Part model, mm, in its own coordinate system. Face numbers are marked on the shaded views. A direction names the side the tool comes from. Give positions to 0.01 mm unless a question says otherwise; leave off trailing zeros. Order: outer loops, then holes, each group sorted by start corner. A loop starts at its lowest first (then second) coordinate and runs counter-clockwise, first axis right, second up. Notation, with made-up numbers: M 67,25 L 104,25 A23 ccw 104,46 Z; hole C 82.5,57.5 d11. An arc over 180 degrees is marked long. Return JSON: item names as keys, results as strings.
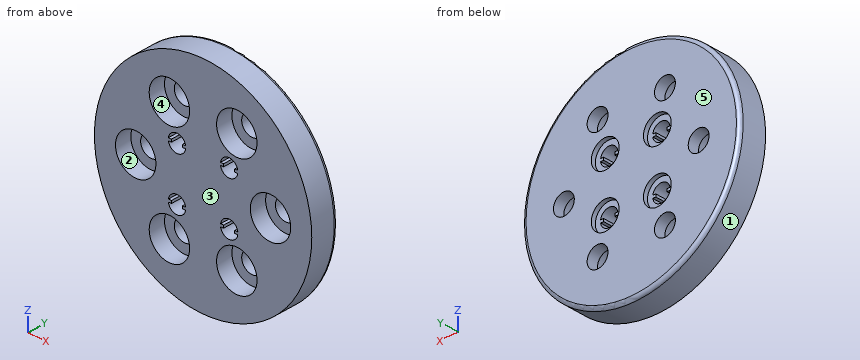
from build123d import *

# Parameters (mm, degrees)
SKETCH1_R           = 25
BOSS_EXTRUDE1_DEPTH = 6.35
SKETCH3_R           = 2.4
CUT_EXTRUDE3_DEPTH  = 7.35
SKETCH4_R           = 4.65
CUT_EXTRUDE4_DEPTH  = 3.8
CIRPATTERN3_COUNT   = 6
SKETCH5_R           = 1.25
CUT_EXTRUDE5_DEPTH  = 7.35
CUT_EXTRUDE6_DEPTH  = 7.35
SKETCH8_R           = 3.2
CUT_EXTRUDE7_DEPTH  = 1
FILLET1_R           = 0.8


with BuildPart() as part:
    # Sketch1 → Boss-Extrude1 (new body)
    with BuildSketch(Plane(origin=(0, 0, 0), x_dir=(1, 0, 0), z_dir=(0, 1, 0))):
        Circle(SKETCH1_R)
    extrude(amount=BOSS_EXTRUDE1_DEPTH)

    # Sketch3 → Cut-Extrude3 (cut, through all)
    with BuildSketch(Plane.XZ):
        with Locations((-15.5, 0)):
            Circle(SKETCH3_R)
    cut_extrude3 = extrude(amount=-CUT_EXTRUDE3_DEPTH, mode=Mode.SUBTRACT)

    # Sketch4 → Cut-Extrude4 (cut)
    with BuildSketch(Plane.XZ):
        with Locations((-15.5, 0)):
            Circle(SKETCH4_R)
    cut_extrude4 = extrude(amount=-CUT_EXTRUDE4_DEPTH, mode=Mode.SUBTRACT)

    # CirPattern3: Cut-Extrude3, Cut-Extrude4 ×6 about axis
    cirpattern3_axis = Axis((0, 0, 0), (0, 1, 0))
    for i in range(1, CIRPATTERN3_COUNT):
        add(cut_extrude3.rotate(cirpattern3_axis, i * 360 / CIRPATTERN3_COUNT), mode=Mode.SUBTRACT)
        add(cut_extrude4.rotate(cirpattern3_axis, i * 360 / CIRPATTERN3_COUNT), mode=Mode.SUBTRACT)

    # Sketch5 → Cut-Extrude5 (cut, through all)
    with BuildSketch(Plane.XZ):
        with Locations((-6, -6)):
            Circle(SKETCH5_R)
        with Locations((6, -6)):
            Circle(SKETCH5_R)
        with Locations((-6, 6)):
            Circle(SKETCH5_R)
        with Locations((6, 6)):
            Circle(SKETCH5_R)
    extrude(amount=-CUT_EXTRUDE5_DEPTH, mode=Mode.SUBTRACT)

    # Sketch7 → Cut-Extrude6 (cut, through all)
    with BuildSketch(Plane(origin=(0, 6.35, 0), x_dir=(1, 0, 0), z_dir=(0, 1, 0))):
        with BuildLine():
            Line((4.022628007, 6.3), (4.722628007, 6.3))
            Line((4.722628007, 6.3), (4.722628007, 5.7))
            Line((4.722628007, 5.7), (4.022628007, 5.7))
            ThreePointArc((4.022628007, 5.7), (6, 4), (7.977371993, 5.7))
            Line((7.977371993, 5.7), (7.277371993, 5.7))
            Line((7.277371993, 5.7), (7.277371993, 6.3))
            Line((7.277371993, 6.3), (7.977371993, 6.3))
            ThreePointArc((7.977371993, 6.3), (6, 8), (4.022628007, 6.3))
        make_face()
        with BuildLine():
            Line((-7.277371993, 6.3), (-7.277371993, 5.7))
            Line((-7.277371993, 5.7), (-7.977371993, 5.7))
            ThreePointArc((-7.977371993, 5.7), (-6, 4), (-4.022628007, 5.7))
            Line((-4.022628007, 5.7), (-4.722628007, 5.7))
            Line((-4.722628007, 5.7), (-4.722628007, 6.3))
            Line((-4.722628007, 6.3), (-4.022628007, 6.3))
            ThreePointArc((-4.022628007, 6.3), (-6, 8), (-7.977371993, 6.3))
            Line((-7.977371993, 6.3), (-7.277371993, 6.3))
        make_face()
        with BuildLine():
            Line((-4.022628007, -6.3), (-4.722628007, -6.3))
            Line((-4.722628007, -6.3), (-4.722628007, -5.7))
            Line((-4.722628007, -5.7), (-4.022628007, -5.7))
            ThreePointArc((-4.022628007, -5.7), (-6, -4), (-7.977371993, -5.7))
            Line((-7.977371993, -5.7), (-7.277371993, -5.7))
            Line((-7.277371993, -5.7), (-7.277371993, -6.3))
            Line((-7.277371993, -6.3), (-7.977371993, -6.3))
            ThreePointArc((-7.977371993, -6.3), (-6, -8), (-4.022628007, -6.3))
        make_face()
        with BuildLine():
            Line((7.277371993, -6.3), (7.277371993, -5.7))
            Line((7.277371993, -5.7), (7.977371993, -5.7))
            ThreePointArc((7.977371993, -5.7), (6, -4), (4.022628007, -5.7))
            Line((4.022628007, -5.7), (4.722628007, -5.7))
            Line((4.722628007, -5.7), (4.722628007, -6.3))
            Line((4.722628007, -6.3), (4.022628007, -6.3))
            ThreePointArc((4.022628007, -6.3), (6, -8), (7.977371993, -6.3))
            Line((7.977371993, -6.3), (7.277371993, -6.3))
        make_face()
    extrude(amount=-CUT_EXTRUDE6_DEPTH, mode=Mode.SUBTRACT)

    # Sketch8 → Cut-Extrude7 (cut)
    with BuildSketch(Plane(origin=(0, 6.35, 0), x_dir=(1, 0, 0), z_dir=(0, 1, 0))):
        with Locations((6, -6)):
            Circle(SKETCH8_R)
        with Locations((6, 6)):
            Circle(SKETCH8_R)
        with Locations((-6, 6)):
            Circle(SKETCH8_R)
        with Locations((-6, -6)):
            Circle(SKETCH8_R)
    extrude(amount=-CUT_EXTRUDE7_DEPTH, mode=Mode.SUBTRACT)

    # Fillet1
    fillet1_edges = [part.edges().sort_by_distance(p)[0] for p in [
        (-25, 6.35, 0),
    ]]
    fillet(fillet1_edges, radius=FILLET1_R)


solid = part.part
Q1. Pin check, flat tips, straight feed: pin 1 (0.8 mm diameter, centred on x = -7.5, y = 2.5, fed in from -Z); pin 2 (4 mm diameter, centred on x = -7.75, z = 13.42, fed in from +Y); pin 3 (0.7 mm diameter, centred on y = 3.5, z = 6, fed in from +X); pin 4 (3 mm diameter, centred on y = 5, z = 13.5, fed in from -X). Stop position of each tip, or through.
Established:
{"pin 1": "stops at z = -23.97", "pin 2": "passes through", "pin 3": "stops at x = 24.35", "pin 4": "stops at x = -21.93"}
Q2. Probe line 1 along Z through (x, y) = (-6, 6); line 2 along X through (y, z) = (6.25, 14); line 3 along Z through (x, y) = (-6, 5.25). List the from-to ranges inside material, lowest first.
Established:
{"line 1": "z = -24.13 to -15.07, -11.78 to -9.2, -2.8 to 2.8, 9.2 to 11.78, 15.07 to 24.13", "line 2": "x = -20.21 to -10.08, -5.42 to 5.42, 10.08 to 20.21", "line 3": "z = -24.27 to -15.07, -11.78 to -8, -4 to 4, 8 to 11.78, 15.07 to 24.27"}
Q3. Band-saw the part on A-A (z = 0). Give the cut face in (x, y).
Established:
{"outline": "M -25,0 L -20.15,0 L -20.15,3.8 L -17.9,3.8 L -17.9,6.35 L -24.2,6.35 A0.8 ccw -25,5.55 Z; M -13.1,3.8 L -10.85,3.8 L -10.85,0 L 10.85,0 L 10.85,3.8 L 13.1,3.8 L 13.1,6.35 L -13.1,6.35 Z; M 17.9,3.8 L 20.15,3.8 L 20.15,0 L 25,0 L 25,5.55 A0.8 ccw 24.2,6.35 L 17.9,6.35 Z"}
Q4. Band-saw the part on B-B (y = 4.5). Give the number of separate pieces and of enclosed holes in the cut face, then the cut area to 3 significant figures.
Established:
{"separate pieces": "1", "enclosed holes": "10", "area": "1,810 mm²"}
Q5. 3-axis set-ups, long thin cutter, end or side, ignore diameter. For the marked faces 4 and 5: which of +Z, -Z, +X, -X, +Y, -Y reach the whole face in a straight line?
Established:
{"face 4": "-Y", "face 5": "+Z, -Z, +X, -X, +Y"}
Q6. Two-plate mould, pull along X, no slides. Class the marked faces 1, 2 and 3: +X half, -X half, draft (parallel to the pull), parting line (faces both ways), or undercut.
Established:
{"face 1": "parting line", "face 2": "undercut", "face 3": "draft"}
